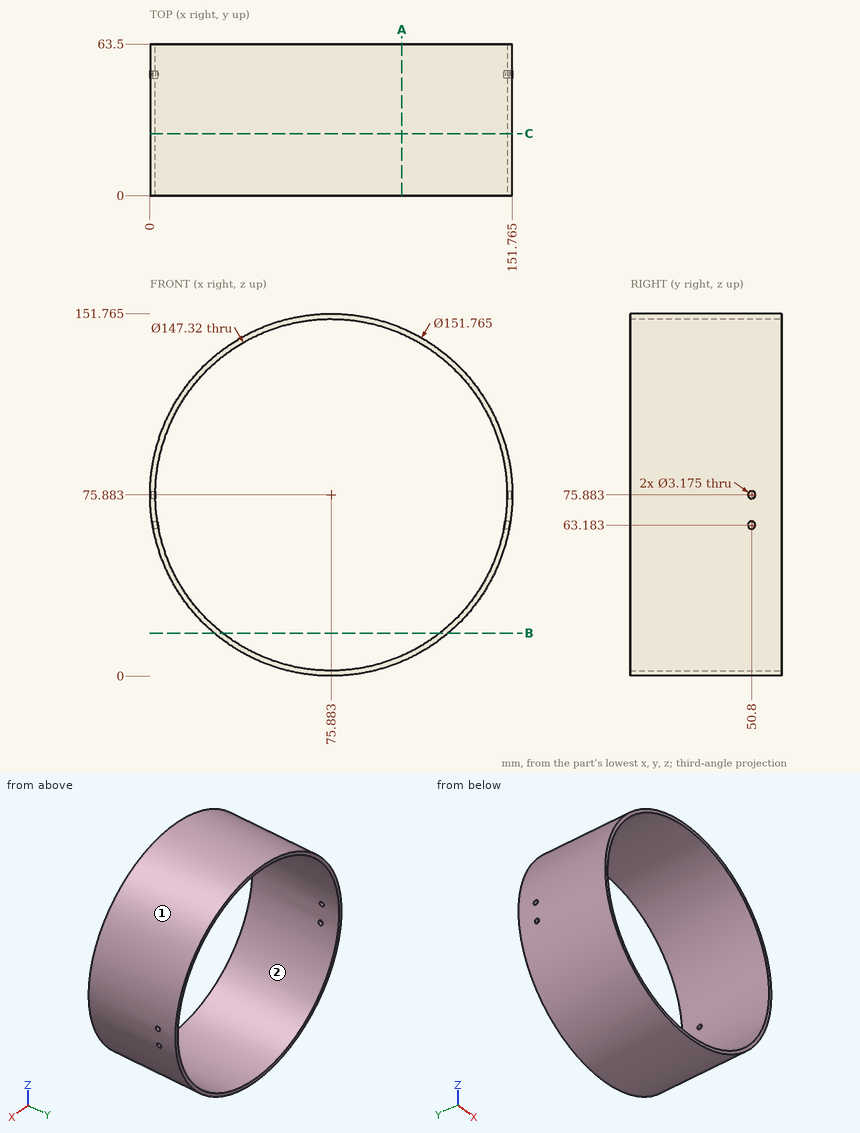
Here's the drawing with two shaded views (mm, measured from the low corner). I have some questions. Give positions to 0.01 mm unless a question says otherwise; leave off trailing zeros. Order: outer loops, then holes, each group sorted by start corner. A loop starts at its lowest first (then second) coordinate and runs counter-clockwise, first axis right, second up. Notation, with made-up numbers: (27.5, -3) - (75.5, -3) arc R14 ccw to (75.5, 14) - close; hole circle Ø8 at (14, -26.5). An arc over 180 degrees is marked (long way). Write each question's results on one line, items separated by ' | '.
1) Please list where these lines run through material, in increasing order: line 1 along Z through (x, y) = (78, 15.5) (1 decimal); line 2 along Z through (x, y) = (66, 15) (1 decimal); line 3 along X through (y, z) = (27.5, 44.5) (1 decimal). Write a range as [from, to].
Final values:
line 1: z = [0, 2.3], [149.5, 151.7] | line 2: z = [0.6, 2.9], [148.9, 151.1] | line 3: x = [6.8, 9.2], [142.5, 145]
2) Suppose I cut it at B-B, the plane z = 18. Write out the boundary of the cut face in (x, y) (1 decimal), then the cut area to 3 significant figures.
Final values:
outline: (26.8, 0) - (30.3, 0) - (30.3, 63.5) - (26.8, 63.5) - close; (121.4, 0) - (125, 0) - (125, 63.5) - (121.4, 63.5) - close | area: 446 mm^2
3) I'm going to push flat-ended pins straight in: pin 1 Ø4 at (y, z) = (50.8, 63.18) entering from +X; pin 2 Ø2 at (x, y) = (133, 31.5) entering from -Z (1 decimal); pin 3 Ø4 at (y, z) = (50.8, 63.18) entering from -X. Where does each tip first touch, or does it pass through?
Final values:
pin 1: stops at x = 151.01 | pin 2: stops at z = 24.8 | pin 3: stops at x = 0.76
4) If we mould it in two halves opening along Z, with no side actions, what happens to the marked faces 1 and 2? For each: pulls with the +Z half, pulls with the -Z half, needs draft (parallel to the pull), parting line crosses it, or undercut.
Final values:
face 1: parting line crosses it | face 2: undercut
5) Suppose I cut it at C-C, the plane y = 26. Write out the boundary of the cut face in (x, z) (1 decimal).
Final values:
outline: circle Ø151.8 at (75.9, 75.9); hole circle Ø147.3 at (75.9, 75.9)
6) Suppose I cut it at A-A, the plane x = 105.5. Write out the boundary of the cut face in (y, z) (1 decimal).
Final values:
outline: (0, 6) - (63.5, 6) - (63.5, 8.4) - (0, 8.4) - close; (0, 143.3) - (63.5, 143.3) - (63.5, 145.7) - (0, 145.7) - close
